Model file for the job. Use its own axes, mm. A direction names the side the tool comes from. Round coordinates to 2 decimals unless told otherwise and drop trailing zeros. Order: outer loops, then holes, each group sorted by start corner. A loop starts at its lowest first (then second) coordinate and runs counter-clockwise, first axis right, second up. Notation, with made-up numbers: (27.5, -29.75) -> (47.5, -29.75) arc R22 ccw to (47.5, -4.75) -> close; hole circle Ø11 at (0.5, 33.5). An arc over 180 degrees is marked (long way). Answer as CSV lines item,"result".
```python
from build123d import *

# Parameters (mm, degrees)
ESQUISSE1_R        = 3.25
ESQUISSE1_R_2      = 3.5
BOSS_EXTRU_1_DEPTH = 10
CONG_1_R           = 6
CONG_2_R           = 8
CONG_3_R           = 7
CONG_4_R           = 2


with BuildPart() as part:
    # Esquisse1 → Boss.-Extru.1 (new body)
    with BuildSketch(Plane.XY):
        Polygon((24, 110), (24, 36), (0, 36), (0, 30), (14, 30), (16.721324328, 16), (34, 16), (34, 110), align=None)
        with Locations((29, 104)):
            Circle(ESQUISSE1_R, mode=Mode.SUBTRACT)
        with Locations((22, 23)):
            Circle(ESQUISSE1_R_2, mode=Mode.SUBTRACT)
        with Locations((29, 87)):
            Circle(ESQUISSE1_R, mode=Mode.SUBTRACT)
        with Locations((29, 70)):
            Circle(ESQUISSE1_R, mode=Mode.SUBTRACT)
        with Locations((29, 53)):
            Circle(ESQUISSE1_R, mode=Mode.SUBTRACT)
    boss_extru_1 = extrude(amount=BOSS_EXTRU_1_DEPTH)

    # Symétrie2: Boss.-Extru.1 across plane
    add(boss_extru_1.mirror(Plane(origin=(0, 36, 10), x_dir=(0, 0, 1), z_dir=(1, 0, 0))))

    # Congé1
    cong_1_edges = [part.edges().sort_by_distance(p)[0] for p in [
        (16.721324328, 16, 5),
        (14, 30, 5),
        (-14, 30, 5),
        (-16.721324328, 16, 5),
    ]]
    fillet(cong_1_edges, radius=CONG_1_R)

    # Congé2
    cong_2_edges = [part.edges().sort_by_distance(p)[0] for p in [
        (34, 16, 5),
        (-34, 16, 5),
    ]]
    fillet(cong_2_edges, radius=CONG_2_R)

    # Congé3
    cong_3_edges = [part.edges().sort_by_distance(p)[0] for p in [
        (34, 110, 5),
        (-34, 110, 5),
    ]]
    fillet(cong_3_edges, radius=CONG_3_R)

    # Congé4
    cong_4_edges = [part.edges().sort_by_distance(p)[0] for p in [
        (24, 36, 5),
        (-24, 36, 5),
    ]]
    fillet(cong_4_edges, radius=CONG_4_R)


solid = part.part
```
Q1. Saw through at D-D (x = 29.5). Write the cut outline in (y, z).
Checks:
outline,"(16.81, 0) -> (49.79, 0) -> (49.79, 10) -> (16.81, 10) -> close; (56.21, 0) -> (66.79, 0) -> (66.79, 10) -> (56.21, 10) -> close; (73.21, 0) -> (83.79, 0) -> (83.79, 10) -> (73.21, 10) -> close; (90.21, 0) -> (100.79, 0) -> (100.79, 10) -> (90.21, 10) -> close; (107.21, 0) -> (109.54, 0) -> (109.54, 10) -> (107.21, 10) -> close"
Q2. Saw through at B-B (y = 23). Write the cut outline in (x, z).
Checks:
outline,"(-33.94, 0) -> (-25.5, 0) -> (-25.5, 10) -> (-33.94, 10) -> close; (-18.5, 0) -> (-15.36, 0) -> (-15.36, 10) -> (-18.5, 10) -> close; (15.36, 0) -> (18.5, 0) -> (18.5, 10) -> (15.36, 10) -> close; (25.5, 0) -> (33.94, 0) -> (33.94, 10) -> (25.5, 10) -> close"
Q3. Wall check: L1, parallel to X at y = 39.5, z = 0.75; L2, parallel to Y at x = -22, z = 4; L3, parallel to Y at x = 29, z = 2.25. Give the ranges that are in metal, low to high. Write a range as [from, to].
Checks:
L1,"[-34, -24], [24, 34]"
L2,"[16, 19.5], [26.5, 36]"
L3,"[16.58, 49.75], [56.25, 66.75], [73.25, 83.75], [90.25, 100.75], [107.25, 109.71]"
Q4. Saw through at A-A (y = 82.5). Write the cut outline in (x, z).
Checks:
outline,"(-34, 0) -> (-24, 0) -> (-24, 10) -> (-34, 10) -> close; (24, 0) -> (34, 0) -> (34, 10) -> (24, 10) -> close"
Q5. Flat gauge pins, fed straight in: pin 1 (1.5 mm diameter, centred on x = 11.5, z = 5.5, fed in from -Y); pin 2 (3 mm diameter, centred on x = -0.5, z = 6.5, fed in from -Y). Where does each tip first touch, or does it go through?
Checks:
pin 1,"y = 29.08"
pin 2,"y = 30"
Q6. Tool access for faces 5 (the flat face through (-15.355, 23.03, 4.93)), 6 (the flat face through (34, 63, 5)): list every direction of +Z, -Z, +X, -X, +Y, -Y with a clear straight run to the whole face (end or side of a thin tool).
Checks:
face 5,"+Z, -Z, -Y"
face 6,"+Z, -Z, +X, +Y, -Y"
Q7. Saw through at C-C (z = 2.75). State how many separate pieces and enclosed holes the cut face has, plus the area to 3 significant figures.
Checks:
separate pieces,"1"
enclosed holes,"10"
area,"2,020 mm²"
Q8. Mould opens along Y. For faces 1 (the flat face through (-34, 63, 5)), 2 (the flat face through (0, 36, 5)), 3 (the cylindrical face through (-12.915, 28.593, 5.07)), 4 (the cylindrical face through (-32.002, 51.755, 4.93)) say: +Y half, -Y half, draft (parallel to the pull), parting line (faces both ways), or undercut.
Checks:
face 1,"draft"
face 2,"+Y half"
face 3,"-Y half"
face 4,"undercut"
